```python
from build123d import *

# Parameters (mm, degrees)
SKETCH_1_R             = 5.5
EXTRUDE_1_DEPTH        = 74
CHAMFER_1_SIZE         = 0.5
SKETCH_2_R             = 3.3
EXTRUDE_2_DEPTH        = 8
HOLE_WIZARD_M5_1_D     = 4.2
HOLE_WIZARD_M5_1_DEPTH = 12.4
HOLE_WIZARD_M5_1_TIP   = 1.2618073
CHAMFER_3_SIZE         = 0.5
SKETCH_6_W             = 10
SKETCH_6_H             = 3
CUT_EXTRUDE_1_DEPTH    = 13


# Read off the part's stored shape, not the designer's step: M6 机械螺纹 螺柱1
with BuildPart() as part:
    # 草图1 → 拉伸1 (new body)
    with BuildSketch(Plane.XY):
        Circle(SKETCH_1_R)
    extrude(amount=EXTRUDE_1_DEPTH)

    # 倒角1
    chamfer_1_edges = [part.edges().sort_by_distance(p)[0] for p in [
        (-5.5, 0, 0),
        (-5.5, 0, 74),
    ]]
    chamfer(chamfer_1_edges, length=CHAMFER_1_SIZE)

    # 草图2 → 拉伸2 (add)
    with BuildSketch(Plane.XY.offset(74)):
        Circle(SKETCH_2_R)
    extrude(amount=EXTRUDE_2_DEPTH)

    # M5 螺纹孔1
    with Locations(Plane(origin=(0, 0, 0), x_dir=(-1, 0, 0), z_dir=(0, 0, -1))):
        with Locations((0, 0)):
            Hole(HOLE_WIZARD_M5_1_D / 2, depth=HOLE_WIZARD_M5_1_DEPTH)
            with Locations((0, 0, -(HOLE_WIZARD_M5_1_DEPTH + HOLE_WIZARD_M5_1_TIP / 2))):  # 118° drill point
                Cone(0, HOLE_WIZARD_M5_1_D / 2, HOLE_WIZARD_M5_1_TIP, mode=Mode.SUBTRACT)

    # 倒角3
    chamfer_3_edges = [part.edges().sort_by_distance(p)[0] for p in [
        (-2.1, 0, 0),
    ]]
    chamfer(chamfer_3_edges, length=CHAMFER_3_SIZE)

    # 草图6 → 切除-拉伸1 (cut)
    with BuildSketch(Plane(origin=(0, 0, 0), x_dir=(-1, 0, 0), z_dir=(0, 0, -1))):
        with Locations((0, 6.5)):
            Rectangle(SKETCH_6_W, SKETCH_6_H)
        with Locations((0, -6.5)):
            Rectangle(SKETCH_6_W, SKETCH_6_H)
    extrude(amount=-CUT_EXTRUDE_1_DEPTH, mode=Mode.SUBTRACT)

    # M6 机械螺纹 螺柱1 outline → M6 机械螺纹 螺柱1 (revolve, cut)
    with BuildSketch(Plane.XZ):
        Polygon((3.3, 82), (2.4585, 82), (3, 81.4585), (3, 74), (3.3, 74), align=None)
    revolve(axis=Axis((0, 0, 0), (0, 0, 1)), mode=Mode.SUBTRACT)


solid = part.part
```
For this review, take the finished solid that the model builds, in its own axes (mm). A direction names the side the tool comes from. Round coordinates to 2 decimals unless told otherwise and drop trailing zeros. Loops run counter-clockwise (first coordinate to the right, second up) from the corner with the lowest first, then second, coordinate; pieces in that order, holes last.
Q1. Machinability: for faces 1 (the face through (0, 5, 6)), 2 (the face through (-0.1, -3.3, 74)), 3 (the face through (-5.134, 0.113, 0.135)), 4 (the face through (0, -5, 6)), 5 (the face through (5.134, -0.113, 0.135)), which of the approach directions +Z, -Z, +X, -X, +Y, -Y give a long, thin tool a straight path to every point of the face, cutting with its end or side? Answer none if there is none.
Result sheet:
face 1: -Z, +X, -X, +Y
face 2: +Z
face 3: -Z, -X
face 4: -Z, +X, -X, -Y
face 5: -Z, +X
Q2. Mouldability with a two-part tool opening along Y and no side actions: class faces 6 (the face through (2.003, 0.631, 6.533)), 7 (the face through (5.08, -2.11, 36.49)), 8 (the face through (2, -2, 0)) as +Y half, -Y half, draft (parallel to the pull), parting line (faces both ways), or undercut.
Result sheet:
face 6: undercut
face 7: parting line
face 8: draft
Q3. Insertion check: pin 1 Ø5 at (x, z) = (0, 6.5) entering from +Y; pin 2 Ø3 at (y, z) = (-3.5, 45.5) entering from +X; pin 3 Ø1 at (y, z) = (4, 32.5) entering from +X. Each pin has a flat end and moves straight along its axis. Give the tip position at first contact, or say it passes through.
Result sheet:
pin 1: stops at y = 5
pin 2: stops at x = 5.12
pin 3: stops at x = 4.24
Q4. Add section B-B on z = 25.5. Write out the cut boundary in (x, y).
Result sheet:
outline: circle Ø11 at (0, 0)
Q5. To check wall thickness, follow line 1 along Y through (x, z) = (0, 6.5); line 2 along X through (y, z) = (0, 5); line 3 along X through (y, z) = (5, 63). State the ranges of each line that lie inside material, in increasing order.
Result sheet:
line 1: y = -5 to -2.1, 2.1 to 5
line 2: x = -5.5 to -2.1, 2.1 to 5.5
line 3: x = -2.29 to 2.29
Q6. Add section A-A on z = 6.5. Write out the cut boundary in (x, y).
Result sheet:
outline: (-2.29, -5) - (2.29, -5) arc R5.5 ccw to (2.29, 5) - (-2.29, 5) arc R5.5 ccw to start; hole circle Ø4.2 at (0, 0)
